Part print with two shaded views. Sizes in mm from the minimum x, y, z corner. Round coordinates to 2 decimals unless told otherwise and drop trailing zeros. Loops run counter-clockwise (first coordinate to the right, second up) from the corner with the lowest first, then second, coordinate; pieces in that order, holes last. Notation, with made-up numbers: (-2, 79.25) -> (40, 79.25) arc R14 cw to (40, 83.25) -> close; hole circle Ø11 at (87.25, 32.25). An arc over 180 degrees is marked (long way). Use a Markdown table: item, result. Add a question column.
Item 1: Cut at A-A, the plane z = 24.5. List the corners of the cut face in (x, y) (1 decimal).
Item 2: Probe line 1 (X direction, y = 1032, z = 17.5); line 2 (X direction, y = 740, z = 19.5) (1 decimal). List the from-to ranges inside material, lowest first. Write a range as [from, to].
Item 3: Flat gauge pins, fed straight in: pin 1 (9 mm diameter, centred on y = 1148, z = 23, fed in from +X) (3 decimals); pin 2 (3 mm diameter, centred on x = 203, y = 395, fed in from -Z); pin 3 (3 mm diameter, centred on y = 597, z = 18, fed in from +X); pin 4 (12 mm diameter, centred on x = 392, z = 30.5, fed in from +Y) (1 decimal). Where does each tip first touch, or does it go through?
Item 4: Cut at C-C, the plane y = 451. List the corners of the cut face in (x, z), plus the area to 3 significant figures.
Item 5: Cut at B-B, the plane x = 46. List the corners of the cut face in (y, z), plus the area to 3 significant figures.
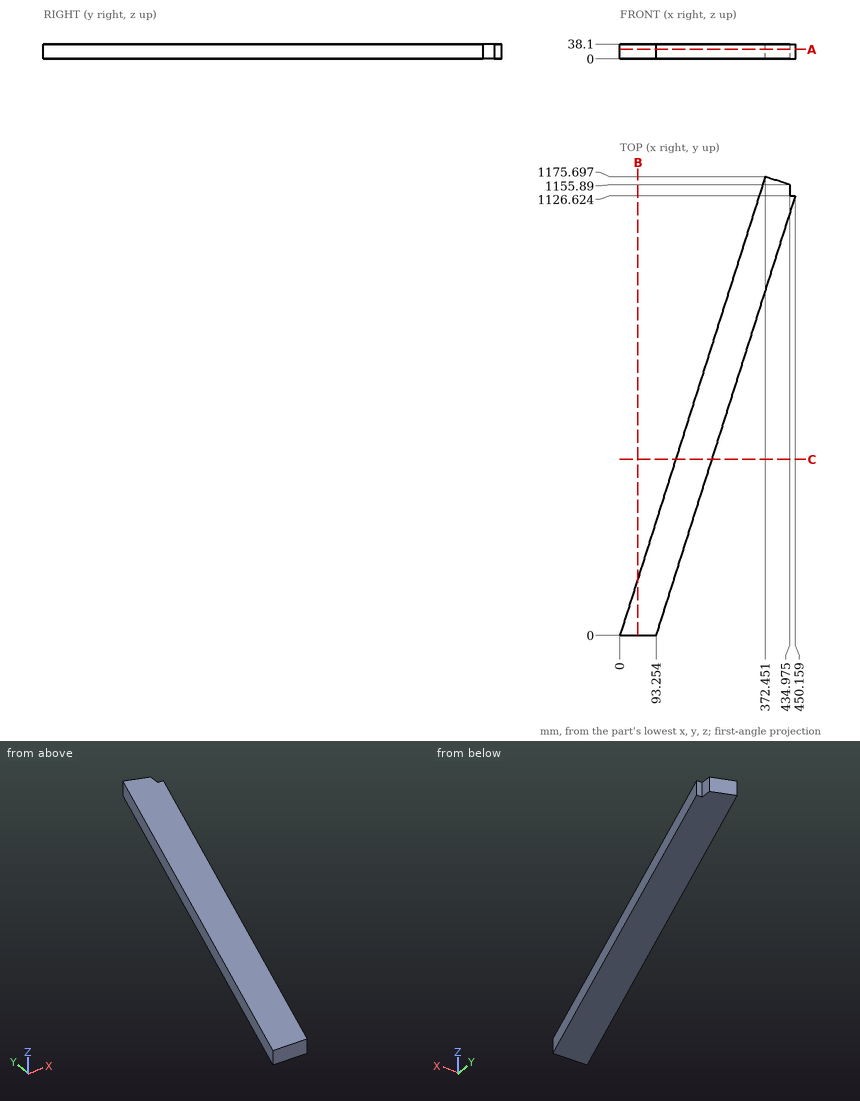
A:
| question | item | result |
|---|---|---|
| 1 | outline | (0, 0) -> (93.3, 0) -> (450.2, 1126.6) -> (435, 1126.6) -> (435, 1155.9) -> (372.5, 1175.7) -> close |
| 2 | line 1 | x = [326.93, 420.18] |
| 2 | line 2 | x = [234.4, 327.7] |
| 3 | pin 1 | stops at x = 434.975 |
| 3 | pin 2 | stops at z = 0 |
| 3 | pin 3 | stops at x = 282.85 |
| 3 | pin 4 | stops at y = 1171.4 |
| 4 | outline | (142.87, 0) -> (236.13, 0) -> (236.13, 38.1) -> (142.87, 38.1) -> close |
| 4 | area | 3,550 mm^2 |
| 5 | outline | (0, 0) -> (145.21, 0) -> (145.21, 38.1) -> (0, 38.1) -> close |
| 5 | area | 5,530 mm^2 |
